Verification items for the finished model (mm, model axes). A direction names the side the tool comes from. Coordinates: 2 decimals unless noted, no trailing zeros. Order: outer loops, then holes, each group sorted by start corner. A loop starts at its lowest first (then second) coordinate and runs counter-clockwise, first axis right, second up. Notation, with made-up numbers: (-15, 3) - (2, 3) arc R22 cw to (2, 26) - close; hole circle Ø7 at (15, -31.75). An arc over 180 degrees is marked (long way). Answer as CSV lines item,"result". Start each with the question number.
1. Section check C-C (x = -83.5). Record the cut outline in (y, z).
2. Mould release check, pull along X, two halves, no side actions. Record for faces 1 (the flat face through (-51, 2, -74.973)), 2 (the flat face through (44.45, 2, -77)), 3 (the flat face through (101.6, 2, 27)), 4 (the flat face through (-58.36, 2.14, 75.08)): pulls with the +X half, pulls with the -X half, needs draft (parallel to the pull), parting line crosses it, or undercut.
3. Go/stop test with flat-tipped pins: pin 1 (1.3 mm diameter, centred on y = 2.5, z = 2, fed in from +X); pin 2 (3 mm diameter, centred on x = 62.5, z = -23, fed in from -Y); pin 3 (1.3 mm diameter, centred on y = 3, z = 0, fed in from -X); pin 4 (2 mm diameter, centred on x = 48.5, y = 3, fed in from -Z). Record where each tip stops, or that it passes through.
4. Set-up check for faces 5 (the flat face through (57.15, 2, -77)), 6 (the flat face through (-97.488, 2, 0)), 7 (the flat face through (-101.6, 2, 28)): record each of +Z, -Z, +X, -X, +Y, -Y from which the full face is reachable in a straight line by a thin tool's end or side.
5. Section check B-B (x = -17). Record the cut outline in (y, z).
6. Material ranges on L1, parallel to X at y = 2.75, z = 6.5; L2, parallel to Z at x = -5.5, y = 2.5; L3, parallel to Z at x = 11.5, y = 1.7, recorded low to high. Write a range as [from, to].
from build123d import *

# Parameters (mm, degrees)
F0_W     = 12.7
F0_H     = 4.3434
F1_DEPTH = 4.3434
F2_W     = 4.3434
F2_H     = 12.7
F3_DEPTH = 4.3444
F5_DEPTH = 4.3444


with BuildPart() as f1:
    # F0 (on Front) → F1 (new body)
    with BuildSketch(Plane.XZ):
        Polygon((50.8, 74.088349), (0, 100.27007), (-50.8, 74.088349), (-62.088889, 68.270189), (-101.6, 47.906629), (-101.6, -79.093371), (-57.15, -79.093371), (-57.15, -74.749971), (-44.45, -74.749971), (-44.45, -79.093371), (44.45, -79.093371), (44.45, -74.749971), (57.15, -74.749971), (57.15, -79.093371), (101.6, -79.093371), (101.6, 47.906629), (62.088889, 68.270189), align=None)
        Polygon((-62.088889, 68.270189), (-50.8, 74.088349), (-52.789811, 77.949149), (-64.0787, 72.130989), align=None)
        Polygon((52.789811, 77.949149), (50.8, 74.088349), (62.088889, 68.270189), (64.0787, 72.130989), align=None)
        with Locations((-50.8, -76.921671)):
            Rectangle(F0_W, F0_H)
        Polygon((50.8, -79.093371), (57.15, -79.093371), (57.15, -74.749971), (44.45, -74.749971), (44.45, -79.093371), align=None)
    extrude(amount=-F1_DEPTH)

    # F2 (on Front) → F3 (cut, through all)
    with BuildSketch(Plane.XZ):
        with Locations((-99.660009, 0.220258)):
            Rectangle(F2_W, F2_H)
        with Locations((99.660009, 0.220258)):
            Rectangle(F2_W, F2_H)
    extrude(amount=-F3_DEPTH, mode=Mode.SUBTRACT)

    # F4 (on Front) → F5 (cut, through all)
    with BuildSketch(Plane.XZ):
        Polygon((-57.15, -79.316832), (-50.8, -79.316832), (-44.45, -79.316832), (-44.45, -74.973432), (-50.8, -74.973432), (-57.15, -74.973432), align=None)
        Polygon((57.15, -79.316832), (57.15, -74.973432), (50.8, -74.973432), (44.45, -74.973432), (44.45, -79.316832), (50.8, -79.316832), align=None)
    extrude(amount=-F5_DEPTH, mode=Mode.SUBTRACT)


solid = f1.part
Evaluation:
1,outline,"(0, -79.09) - (4.34, -79.09) - (4.34, 57.24) - (0, 57.24) - close"
2,face 1,"undercut"
2,face 2,"undercut"
2,face 3,"pulls with the +X half"
2,face 4,"pulls with the -X half"
3,pin 1,"stops at x = 97.49"
3,pin 2,"stops at y = 0"
3,pin 3,"stops at x = -97.49"
3,pin 4,"stops at z = -74.97"
4,face 5,"-Z, +Y, -Y"
4,face 6,"-X, +Y, -Y"
4,face 7,"+Z, -Z, -X, +Y, -Y"
5,outline,"(0, -79.09) - (4.34, -79.09) - (4.34, 91.51) - (0, 91.51) - close"
6,L1,"x = [-97.49, 97.49]"
6,L2,"z = [-79.09, 97.44]"
6,L3,"z = [-79.09, 94.34]"
